Autodesk Inventor part; units mm, degrees
ref_plane "YZ Plane" through (0, 0, 0) normal (1, 0, 0) x (0, 1, 0)
ref_plane "XZ Plane" through (0, 0, 0) normal (0, 1, 0) x (-1, 0, 0)
ref_plane "XY Plane" through (0, 0, 0) normal (0, 0, 1) x (1, 0, 0)
sketch "Эскиз1" plane through (0, 0, 0) normal (0, 0, 1) x (1, 0, 0)
  circle A0 centre (0, 0) radius 5
  dimension "d0" = 10
extrude "Выдавливание1" add sketch "Эскиз1" along normal blind 8
sketch "Эскиз2" plane through (0, 0, 8) normal (0, 0, 1) x (1, 0, 0)
  line L0 (0, 0) -> (0, 1.8)
  circle A0 centre (0, 1.8) radius 1
  dimension "d3" = 1.8
  dimension "d4" = 2
extrude "Выдавливание2" add sketch "Эскиз2" along normal blind 7
sketch "Sketch3" plane through (0, 0, 0) normal (0, 0, -1) x (-1, 0, 0)
  circle A0 centre (0, 0) radius 1.55
  dimension "d7" = 3.1
extrude "Extrusion3" cut sketch "Sketch3" against normal blind 6
fillet "Fillet1" radius 1 1 edges at (-1, 1.8, 8)
properties part number "excentrick_2" material "Stainless Steel"
Work out the finished part from the listing and answer in its coordinate system (mm). Give positions to 0.01 mm unless a question says otherwise; leave off trailing zeros. Order: outer loops, then holes, each group sorted by start corner. A loop starts at its lowest first (then second) coordinate and runs counter-clockwise, first axis right, second up. Notation, with made-up numbers: M 71.5,-17.75 L 117.5,-17.75 A9 ccw 117.5,-2.75 Z; hole C -20.5,26.25 d1. An arc over 180 degrees is marked long. Return JSON: item names as keys, results as strings.
1) Each of these flat-tipped pins is pushed along its axis until it touches: pin 1 (1.5 mm diameter, centred on x = 1, z = 12, fed in from -Y); pin 2 (5 mm diameter, centred on x = 0, z = 13.5, fed in from +Y). Where does it stop, or does it pass through?
Resolved:
{"pin 1": "y = 0.83", "pin 2": "y = 2.8"}
2) Section C-C, the plane z = 1 is taken. Write down the section's boundary in (x, y), plus the area to 3 significant figures.
Resolved:
{"outline": "C 0,0 d10; hole C 0,0 d3.1", "area": "71.0 mm^2"}
3) Section A-A, the plane x = 0 is taken. Write down the section's boundary in (y, z).
Resolved:
{"outline": "M -5,0 L -1.55,0 L -1.55,6 L 1.55,6 L 1.55,0 L 5,0 L 5,8 L 3.8,8 A1 cw 2.8,9 L 2.8,15 L 0.8,15 L 0.8,9 A1 cw -0.2,8 L -5,8 Z"}
4) Section D-D, the plane z = 7 is taken. Write down the section's boundary in (x, y), plus the area to 3 significant figures.
Resolved:
{"outline": "C 0,0 d10", "area": "78.5 mm^2"}
5) For a pull along Y with two mould halves and no side action, classify faces 1 (the cylindrical face through (-0.217, 2.776, 11.958)), 2 (the flat face through (0, 0, 6)), 3 (the cylindrical face through (-0.715, -1.375, 2.958)), 4 (the flat face through (0, -1, 8)) as +Y half, -Y half, draft (parallel to the pull), parting line (faces both ways), or undercut.
Resolved:
{"face 1": "parting line", "face 2": "undercut", "face 3": "undercut", "face 4": "draft"}
6) Straight lines are drawn through the part: line 1 along Y through (x, z) = (0, 3.7); line 2 along Z through (x, y) = (0.25, -3.5); line 3 along Y through (x, z) = (0, 9.5). For each, find the intervals that lie inside material, in ascending order. Write a range as [from, to].
Resolved:
{"line 1": "[-5, -1.55], [1.55, 5]", "line 2": "[0, 8]", "line 3": "[0.8, 2.8]"}
7) Section B-B, the plane y = 1.8 is taken. Write down the section's boundary in (x, z), plus the area to 3 significant figures.
Resolved:
{"outline": "M -4.66,0 L 4.66,0 L 4.66,8 L 2,8 A1 cw 1,9 L 1,15 L -1,15 L -1,9 A1 cw -2,8 L -4.66,8 Z", "area": "89.1 mm^2"}
